Check sheet for the modelled part. Datum: model origin and axes. Units: mm. A direction names the side the tool comes from. Coordinates: 2 decimals unless noted, no trailing zeros. Loops run counter-clockwise (first coordinate to the right, second up) from the corner with the lowest first, then second, coordinate; pieces in that order, holes last. Notation, with made-up numbers: (86, 71) -> (143, 71) arc R16 ccw to (143, 95) -> close; hole circle Ø11 at (46, -12). An arc over 180 degrees is marked (long way). Use CSV: the item, a comma, the result in double quotes. Start each with the question number.
1. Thickness scan on L1, parallel to Z at x = 4.75, y = 11.25; L2, parallel to X at y = 10.25, z = 15; L3, parallel to Y at x = 17, z = -13.5. Record the ranges inside material, lowest first.
2. Set-up check for faces 1 (the face through (2.72, -5.05, 24.93)), 2 (the face through (25.393, 0, 5)), 3 (the face through (1.056, 4.018, -19.72)): record each of +Z, -Z, +X, -X, +Y, -Y from which the full face is reachable in a straight line by a thin tool's end or side.
3. Sectioned sample at D-D, the plane z = -33. Record the cut outline in (x, y).
4. Release check for a two-part mould opening along Z. For faces 4 (the face through (11, 1, 30)), 5 (the face through (20.234, 3.997, 14.93)), 6 (the face through (-0.641, -10.613, 4.93)) record: pulls with the +Z half, pulls with the -Z half, needs draft (parallel to the pull), parting line crosses it, or undercut.
5. Gauge pin test, flat ends, axial feed: pin 1 (2 mm diameter, centred on x = 2.5, z = -25.5, fed in from +Y); pin 2 (3 mm diameter, centred on y = -4, z = -29.5, fed in from -X); pin 3 (4 mm diameter, centred on x = 15.5, y = 13, fed in from -Z). Record the tip position at first contact, or that the pin passes through.
6. Sectioned sample at C-C, the plane z = 12. Record the cut outline in (x, y).
```python
from build123d import *

# Parameters (mm, degrees)
BOSS_EXTRUDE1_DEPTH = 10
SKETCH2_R           = 10
BOSS_EXTRUDE2_DEPTH = 10
SKETCH3_R           = 10
BOSS_EXTRUDE3_DEPTH = 10
SKETCH4_R           = 9.92496084
BOSS_EXTRUDE4_DEPTH = 40


with BuildPart() as part:
    # Sketch1 → Boss-Extrude1 (new body)
    with BuildSketch(Plane.XY):
        Polygon((3.215110596, 16.166425121), (19.120786924, 16.166425121), (25.392646828, 6.257971014), (25.392646828, -7.300966184), (19.120786924, -13.833574879), (3.215110596, -13.833574879), (-4.607353172, -7.300966184), (-4.607353172, 6.257971014), align=None)
    extrude(amount=BOSS_EXTRUDE1_DEPTH)

    # Sketch2 → Boss-Extrude2 (add)
    with BuildSketch(Plane.XY.offset(10)):
        with Locations((10.695865166, 0.993157499)):
            Circle(SKETCH2_R)
    extrude(amount=BOSS_EXTRUDE2_DEPTH)

    # Sketch3 → Boss-Extrude3 (add)
    with BuildSketch(Plane.XY.offset(20)):
        with Locations((10.65254826, 1.036474405)):
            Circle(SKETCH3_R)
    extrude(amount=BOSS_EXTRUDE3_DEPTH)

    # Sketch4 → Boss-Extrude4 (add)
    with BuildSketch(Plane(origin=(0, 0, 0), x_dir=(-1, 0, 0), z_dir=(0, 0, -1))):
        with Locations((-10.522597544, 1.036474405)):
            Circle(SKETCH4_R)
    extrude(amount=BOSS_EXTRUDE4_DEPTH)


solid = part.part
```
Completed:
1,L1,"0 to 10"
1,L2,"6.91 to 14.48"
1,L3,"-6.48 to 8.56"
2,face 1,"+Z"
2,face 2,"+Z, -Z, +X, +Y, -Y"
2,face 3,"-Z"
3,outline,"circle Ø19.85 at (10.52, 1.04)"
4,face 4,"pulls with the +Z half"
4,face 5,"undercut"
4,face 6,"needs draft"
5,pin 1,"y = 8.05"
5,pin 2,"x = 1.25"
5,pin 3,"z = 0"
6,outline,"circle Ø20 at (10.7, 0.99)"
